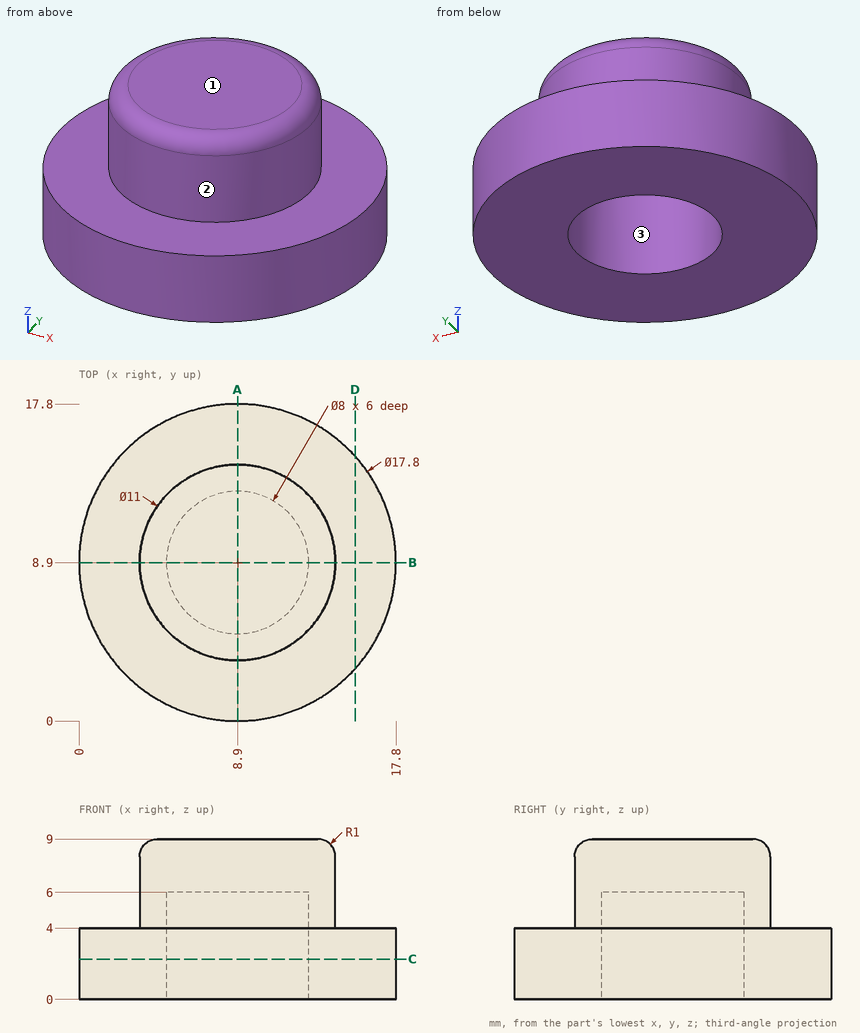
Here's the drawing with two shaded views (mm, measured from the low corner). I have some questions. A direction names the side the tool comes from. Give positions to 0.01 mm unless a question says otherwise; leave off trailing zeros. Loops run counter-clockwise (first coordinate to the right, second up) from the corner with the lowest first, then second, coordinate; pieces in that order, holes last. Notation, with made-up numbers: M 85.25,8 L 129.25,8 A32 cw 129.25,41 Z; hole C -14.5,75 d1. An arc over 180 degrees is marked long. One line per item, written item: value.
(1) Suppose I cut it at C-C on z = 2.25. List the corners of the cut face in (x, y) for me.
Returned:
outline: C 8.9,8.9 d17.8; hole C 8.9,8.9 d8
(2) Suppose I cut it at D-D on x = 15.5. List the corners of the cut face in (y, z) for me.
Returned:
outline: M 2.93,0 L 14.87,0 L 14.87,4 L 2.93,4 Z
(3) Which directions (+Z, -Z, +X, -X, +Y, -Y) give clear straight access to the entire face, cutting with the end or side of a thin tool? Please do the marked faces 1, 2 and 3.
Returned:
face 1: +Z, +X, -X, +Y, -Y
face 2: +Z
face 3: -Z
(4) Will these pins go through, and if not, where does the flat tip stop? pin 1 (3 mm diameter, centred on y = 10, z = 7, fed in from +X); pin 2 (5 mm diameter, centred on x = 10.5, z = 8, fed in from -Y); pin 3 (6.5 mm diameter, centred on x = 9.5, y = 9, fed in from -Z).
Returned:
pin 1: x = 14.4
pin 2: y = 3.4
pin 3: z = 6
(5) Suppose I cut it at A-A on x = 8.9. List the corners of the cut face in (y, z) for me.
Returned:
outline: M 0,0 L 4.9,0 L 4.9,6 L 12.9,6 L 12.9,0 L 17.8,0 L 17.8,4 L 14.4,4 L 14.4,8 A1 ccw 13.4,9 L 4.4,9 A1 ccw 3.4,8 L 3.4,4 L 0,4 Z
(6) I need wall thicknesses on line 1 (Y direction, x = 8.9, z = 1.3); line 2 (Z direction, x = 4.25, y = 12.5); line 3 (X direction, y = 11, z = 4.5). Which ranges of each line are inside material? Lowest first, please.
Returned:
line 1: 0 to 4.9, 12.9 to 17.8
line 2: 0 to 4
line 3: 3.82 to 5.5, 12.3 to 13.98
